Build history of the part. All positions in model axes, mm. Face numbers are marked on the shaded views. Give positions to 0.01 mm unless a question says otherwise; leave off trailing zeros. Order: outer loops, then holes, each group sorted by start corner. A loop starts at its lowest first (then second) coordinate and runs counter-clockwise, first axis right, second up. Notation, with made-up numbers: (-21, 55) - (3, 55) arc R22 cw to (3, 79) - close; hole circle Ø3 at (-39, -9.5). An arc over 180 degrees is marked (long way). Answer in a Markdown table with one row per item.
```python
from build123d import *

# Parameters (mm, degrees)
SKETCH1_R            = 5
BOSS_EXTRUDE1_DEPTH  = 15
M5_CLEARANCE_HOLE1_D = 5.3
CHAMFER1_SIZE        = 0.25


with BuildPart() as part:
    # Sketch1 → Boss-Extrude1 (new, symmetric)
    with BuildSketch(Plane(origin=(0, 0, 0), x_dir=(1, 0, 0), z_dir=(0, 1, 0))):
        with Locations(Location((0, 0, 0), (0, 0, 270))):
            Circle(SKETCH1_R)
    extrude(amount=BOSS_EXTRUDE1_DEPTH, both=True)

    # M5 Clearance Hole1 (through all)
    with Locations(Plane(origin=(0, 15, 0), x_dir=(1, 0, 0), z_dir=(0, 1, 0))):
        with Locations((0, 0)):
            Hole(M5_CLEARANCE_HOLE1_D / 2)

    # Chamfer1
    chamfer1_edges = [part.edges().sort_by_distance(p)[0] for p in [
        (2.65, 15, 0),
        (2.65, -15, 0),
    ]]
    chamfer(chamfer1_edges, length=CHAMFER1_SIZE)


solid = part.part
```
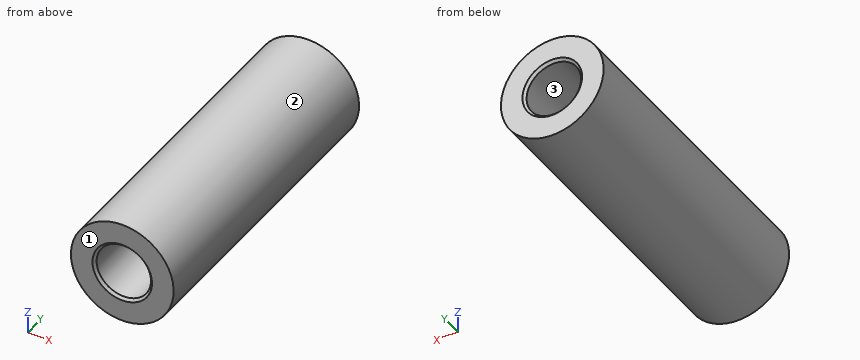
1. Cut at C-C on y = 12.25. Write the cut outline in (x, z), and give its area (3 significant figures).
Check result:
| item | result |
|---|---|
| outline | circle Ø10 at (0, 0); hole circle Ø5.3 at (0, 0) |
| area | 56.5 mm² |
2. Two-plate mould, pull along Z, no slides. Class the marked faces 1, 2 and 3: +Z half, -Z half, draft (parallel to the pull), parting line (faces both ways), or undercut.
Check result:
| item | result |
|---|---|
| face 1 | draft |
| face 2 | parting line |
| face 3 | undercut |
3. Cut at B-B on z = 0. Write the cut outline in (x, y), and give its area (3 significant figures).
Check result:
| item | result |
|---|---|
| outline | (-5, -15) - (-2.9, -15) - (-2.65, -14.75) - (-2.65, 14.75) - (-2.9, 15) - (-5, 15) - close; (2.65, -14.75) - (2.9, -15) - (5, -15) - (5, 15) - (2.9, 15) - (2.65, 14.75) - close |
| area | 141 mm² |
4. Cut at D-D on x = 4. Write the cut outline in (y, z).
Check result:
| item | result |
|---|---|
| outline | (-15, -3) - (15, -3) - (15, 3) - (-15, 3) - close |
5. Probe line 1 (X direction, y = -7.25, z = 0); line 2 (Z direction, x = -2, y = 9); line 3 (X direction, y = 10.5, z = -1.5). List the from-to ranges inside material, lowest first.
Check result:
| item | result |
|---|---|
| line 1 | x = -5 to -2.65, 2.65 to 5 |
| line 2 | z = -4.58 to -1.74, 1.74 to 4.58 |
| line 3 | x = -4.77 to -2.18, 2.18 to 4.77 |
6. Drop flat-ended pins along their axis: P1, Ø3, axis at y = 5, z = -2, coming from the -X side; P2, Ø2, axis at x = 1.5, y = 6, coming from the +Z side; P3, Ø1.5, axis at x = -3.5, y = 5.5, coming from the +Z side. Give the stop position or say it passes through.
Check result:
| item | result |
|---|---|
| P1 | stops at x = -4.97 |
| P2 | stops at z = 4.97 |
| P3 | stops at z = 4.18 |
7. Cut at A-A on x = 0. Write the cut outline in (y, z).
Check result:
| item | result |
|---|---|
| outline | (-15, -5) - (15, -5) - (15, -2.9) - (14.75, -2.65) - (-14.75, -2.65) - (-15, -2.9) - close; (-15, 2.9) - (-14.75, 2.65) - (14.75, 2.65) - (15, 2.9) - (15, 5) - (-15, 5) - close |
